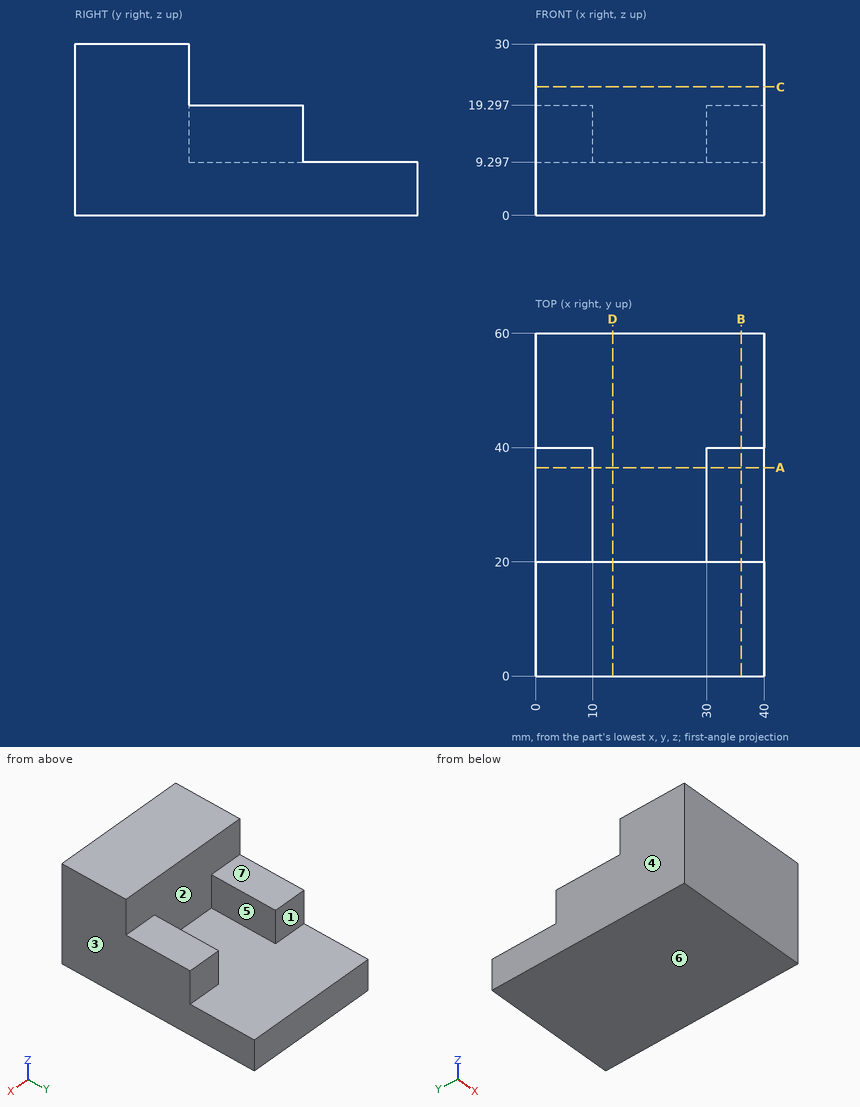
Design review of the part shown in the three views and the two pictorial views. Dimensions are in mm from the part's minimum x, y and z. A direction names the side the tool comes from. Round coordinates to 2 decimals unless told otherwise and drop trailing zeros. Loops run counter-clockwise (first coordinate to the right, second up) from the corner with the lowest first, then second, coordinate; pieces in that order, holes last. Notation, with made-up numbers: (55.25, -17.75) - (84.25, -17.75) arc R31 ccw to (84.25, 17.25) - close; hole circle Ø4 at (24, 32.5). An arc over 180 degrees is marked (long way). Answer as CSV lines item,"result".
(1) Consider section B-B on x = 36. Give the boundary of the cut face in (y, z), then the cut area to 3 significant figures.
Checked values:
outline,"(0, 0) - (60, 0) - (60, 9.3) - (40, 9.3) - (40, 19.3) - (20, 19.3) - (20, 30) - (0, 30) - close"
area,"1,170 mm2"
(2) Insertion check: P1, Ø1.5, axis at x = 15, z = 11.5, coming from the +Y side; P2, Ø3, axis at x = 35.5, y = 28.5, coming from the +Z side; P3, Ø4, axis at x = 18.5, y = 38, coming from the +Z side. Each pin has a flat end and moves straight along its axis. Give the tip position at first contact, or say it passes through.
Checked values:
P1,"stops at y = 20"
P2,"stops at z = 19.3"
P3,"stops at z = 9.3"
(3) Wall thickness on line 1 (X direction, y = 37.5, z = 13.25); line 2 (Z direction, x = 16, y = 42); line 3 (Y direction, x = 18.5, z = 25.5): over which ranges is each line inside the solid? List them lowest first.
Checked values:
line 1,"x = 0 to 10, 30 to 40"
line 2,"z = 0 to 9.3"
line 3,"y = 0 to 20"
(4) Mouldability with a two-part tool opening along X and no side actions: class the marked faces 1, 2, 3 and 4 as +X half, -X half, draft (parallel to the pull), parting line (faces both ways), or undercut.
Checked values:
face 1,"draft"
face 2,"undercut"
face 3,"+X half"
face 4,"-X half"
(5) Consider section A-A on y = 36.5. Give the boundary of the cut face in (x, z).
Checked values:
outline,"(0, 0) - (40, 0) - (40, 19.3) - (30, 19.3) - (30, 9.3) - (10, 9.3) - (10, 19.3) - (0, 19.3) - close"
(6) Consider section C-C on z = 22.5. Give the boundary of the cut face in (x, y), then the cut area to 3 significant figures.
Checked values:
outline,"(0, 0) - (40, 0) - (40, 20) - (0, 20) - close"
area,"800 mm2"
(7) Consider section D-D on x = 13.5. Give the boundary of the cut face in (y, z).
Checked values:
outline,"(0, 0) - (60, 0) - (60, 9.3) - (20, 9.3) - (20, 30) - (0, 30) - close"
(8) Tool access review of the marked faces 5, 6 and 7: name each direction out of +Z, -Z, +X, -X, +Y, -Y from which nothing blocks a thin tool from reaching the whole face with its end or side.
Checked values:
face 5,"+Z, +Y"
face 6,"-Z, +X, -X, +Y, -Y"
face 7,"+Z, +X, -X, +Y"
